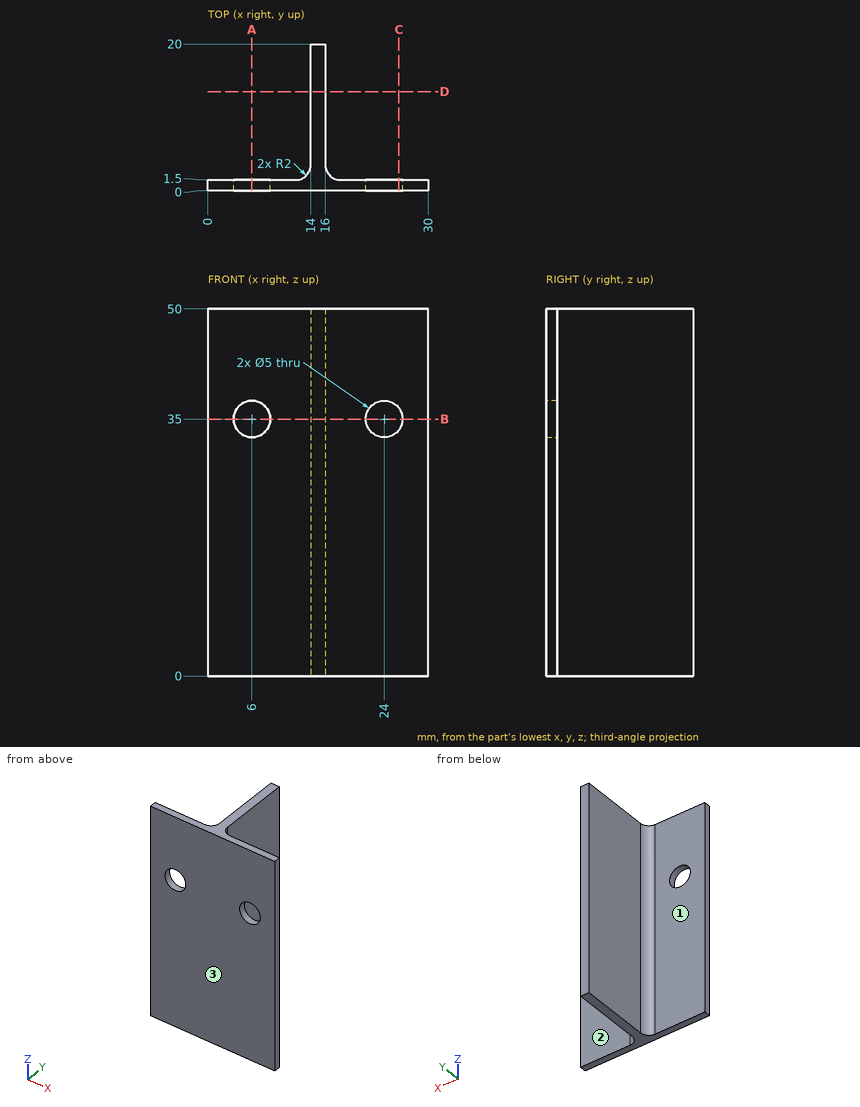
Could you check a few things on this drawing? It's one solid part, dimensions in mm from its lowest x, y, z. A direction names the side the tool comes from. Coordinates: 2 decimals unless noted, no trailing zeros. Order: outer loops, then holes, each group sorted by start corner. A loop starts at its lowest first (then second) coordinate and runs counter-clockwise, first axis right, second up.
1. If we section it at B-B (z = 35): Please give me the cut outline in (x, y), then the cut area to 3 significant figures.
2. For the marked faces 1, 2 and 3, which set-ups out of +Z, -Z, +X, -X, +Y, -Y let a thin tool reach every point of the face, with its end or its side?
3. If we section it at A-A (x = 6): Please give me the cut outline in (y, z).
4. I'm going to push flat-ended pins straight in: pin 1 (4 mm diameter, centred on y = 10.5, z = 12, fed in from -X); pin 2 (6 mm diameter, centred on x = 22.5, z = 21.5, fed in from +Y); pin 3 (6 mm diameter, centred on x = 6, z = 35, fed in from -Y); pin 4 (8 mm diameter, centred on y = 7, z = 26, fed in from -X). Where does each tip first touch, or does it pass through?
5. I need wall thicknesses on line 1 (X direction, y = 0.85, z = 35); line 2 (Y direction, x = 9, z = 15.5); line 3 (X direction, y = 17, z = 9). Which ranges of each line are inside material? Lowest first, please.
6. If we section it at D-D (y = 13.5): Please give me the cut outline in (x, z).
7. If we section it at C-C (x = 26): Please give me the cut outline in (y, z), then the cut area to 3 significant figures.
Entries:
1. outline: (0, 0) - (3.5, 0) - (3.5, 1.5) - (0, 1.5) - close; (8.5, 0) - (21.5, 0) - (21.5, 1.5) - (18, 1.5) arc R2 cw to (16, 3.5) - (16, 20) - (14, 20) - (14, 3.5) arc R2 cw to (12, 1.5) - (8.5, 1.5) - close; (26.5, 0) - (30, 0) - (30, 1.5) - (26.5, 1.5) - close
1. area: 68.7 mm2
2. face 1: +Z, -Z, -X, +Y
2. face 2: +Z, -Z, +X, +Y
2. face 3: +Z, -Z, +X, -X, -Y
3. outline: (0, 0) - (1.5, 0) - (1.5, 32.5) - (0, 32.5) - close; (0, 37.5) - (1.5, 37.5) - (1.5, 50) - (0, 50) - close
4. pin 1: stops at x = 14
4. pin 2: stops at y = 1.5
4. pin 3: stops at y = 0
4. pin 4: stops at x = 13.94
5. line 1: x = 0 to 3.5, 8.5 to 21.5, 26.5 to 30
5. line 2: y = 0 to 1.5
5. line 3: x = 14 to 16
6. outline: (14, 0) - (16, 0) - (16, 50) - (14, 50) - close
7. outline: (0, 0) - (1.5, 0) - (1.5, 33.5) - (0, 33.5) - close; (0, 36.5) - (1.5, 36.5) - (1.5, 50) - (0, 50) - close
7. area: 70.5 mm2
